Design review of the part built by this model. Coordinates are the model's own, in mm. A direction names the side the tool comes from. Round coordinates to 2 decimals unless told otherwise and drop trailing zeros. Write each loop counter-clockwise with the first axis right and the second up, starting at its lowest first coordinate (ties: lowest second). Pieces come first, ordered by that corner, then holes. Notation, with made-up numbers: (18.25, 45.5) -> (53.25, 45.5) arc R21 ccw to (53.25, 66.5) -> close; hole circle Ø9 at (45.5, 72). An arc over 180 degrees is marked (long way). Write item = value, one per line. Start each with the question number.
Item 1: To check wall thickness, follow L1, parallel to X at y = 1, z = -2.5; L2, parallel to X at y = 1.2, z = 18.5; L3, parallel to X at y = 12.5, z = 10.75. State the ranges of each line that lie inside material, in increasing order.
Item 2: Add section D-D, the plane z = 19. State the section outline as (x, y) points.
Item 3: Add section B-B, the plane x = 45.5. State the section outline as (y, z) points, then the cut area to 3 significant figures.
Item 4: For pin 1 Ø2.5 at (x, y) = (29, 4.5) entering from -Z; pin 2 Ø8 at (x, y) = (7, 13) entering from +Z; pin 3 Ø4 at (x, y) = (18, 3) entering from +Z; pin 4 Ø2 at (x, y) = (53.5, 3.5) entering from +Z, all flat-tipped, find the tip position at first contact; note any pin that passes through.
Item 5: Mouldability with a two-part tool opening along X and no side actions: class faces 1 (the cylindrical face through (-0.507, 12.187, 4.774)), 2 (the cylindrical face through (44.036, 0.986, -2.175)), 3 (the flat face through (51, 5.88, 8.08)) as released by +X, released by -X, zero draft, split by the parting line, or undercut.
Item 6: Add section A-A, the plane z = -2.5. State the section outline as (x, y) points, then the cut area to 3 significant figures.
Item 7: Add section C-C, the plane x = 29. State the section outline as (y, z) points, then the cut area to 3 significant figures.
Item 8: Machinability: for faces 4 (the flat face through (0, 1.9, 11.3)), 5 (the flat face through (3, 2, 17)), 6 (the flat face through (42, 1, -3)), 7 (the flat face through (47, 2, -1)), 8 (the cylindrical face through (56.916, 8.056, 7.409)), which of the approach directions +Z, -Z, +X, -X, +Y, -Y give a long, thin tool a straight path to every point of the face, cutting with its end or side? Answer none if there is none.
from build123d import *

# Parameters (mm, degrees)
SKETCH_1_W           = 50
SKETCH_1_H           = 16
EXTRUDE_1_DEPTH      = 15
SKETCH_2_W           = 8
SKETCH_2_H           = 5.2
SKETCH_2_R           = 1.5
EXTRUDE_2_DEPTH      = 2
FILLET_1_R           = 7
EXTRUDE_3_DEPTH      = 1
EXTRUDE_3_DEPTH_BACK = 51
SKETCH_3_R           = 6
EXTRUDE_4_DEPTH      = 12
EXTRUDE_4_DEPTH_BACK = 63
SKETCH_4_R           = 1.1


with BuildPart() as part:
    # Эскиз1 → Бобышка-Вытянуть1 (new body)
    with BuildSketch(Plane(origin=(0, 0, 0), x_dir=(1, 0, 0), z_dir=(0, 1, 0))):
        with Locations((25, -8)):
            Rectangle(SKETCH_1_W, SKETCH_1_H)
    extrude(amount=EXTRUDE_1_DEPTH)

    # Эскиз2 → Бобышка-Вытянуть2 (add)
    # profile 1 of 2: a face of its own
    with BuildSketch(Plane.XZ):
        with Locations((4, 18.6)):
            Rectangle(SKETCH_2_W, SKETCH_2_H)
        with Locations(Location((4.5, 18.5, 0), (0, 0, 270))):
            Circle(SKETCH_2_R, mode=Mode.SUBTRACT)
    # profile 2 of 2: a face of its own
    with BuildSketch(Plane.XZ):
        with Locations((46, -2.6)):
            Rectangle(SKETCH_2_W, SKETCH_2_H)
        with Locations(Location((45.5, -2.5, 0), (0, 0, 270))):
            Circle(SKETCH_2_R, mode=Mode.SUBTRACT)
    extrude(amount=-EXTRUDE_2_DEPTH)

    # Скругление1
    fillet_1_edges = [part.edges().sort_by_distance(p)[0] for p in [
        (25, 15, 0),
        (25, 15, 16),
    ]]
    fillet(fillet_1_edges, radius=FILLET_1_R)

    # Эскиз3 → Бобышка-Вытянуть3 (add, two sides: drawn at the far end of the back side and taken through both)
    with BuildSketch(Plane(origin=(50, 0, 0), x_dir=(0, 0, -1), z_dir=(1, 0, 0)).offset(-EXTRUDE_3_DEPTH_BACK)):
        with Locations((-8, 7.128166943)):
            Circle(SKETCH_3_R)
    extrude(amount=EXTRUDE_3_DEPTH + EXTRUDE_3_DEPTH_BACK)

    # Эскиз4 → Бобышка-Вытянуть4 (add, two sides: drawn at the far end of the back side and taken through both)
    with BuildSketch(Plane(origin=(51, 0, 0), x_dir=(0, 0, -1), z_dir=(1, 0, 0)).offset(-EXTRUDE_4_DEPTH_BACK)):
        with Locations((-8, 7.128166943)):
            Circle(SKETCH_4_R)
    extrude(amount=EXTRUDE_4_DEPTH + EXTRUDE_4_DEPTH_BACK)


solid = part.part
Result set:
q1.L1 = 42 to 44, 47 to 50
q1.L2 = 0 to 3, 6 to 8
q1.L3 = 0 to 50
q2.outline = (0, 0) -> (3.09, 0) -> (3.09, 2) -> (0, 2) -> close; (5.91, 0) -> (8, 0) -> (8, 2) -> (5.91, 2) -> close
q3.outline = (0, -5.2) -> (2, -5.2) -> (2, -4) -> (0, -4) -> close; (0, -1) -> (2, -1) -> (2, 0) -> (8, 0) arc R7 ccw to (15, 7) -> (15, 9) arc R7 ccw to (8, 16) -> (0, 16) -> close
q3.area = 223 mm²
q4.pin_1 = 0
q4.pin_2 = 15.93
q4.pin_3 = 16
q4.pin_4 = through
q5.face_1 = zero draft
q5.face_2 = undercut
q5.face_3 = released by +X
q6.outline = (42, 0) -> (44, 0) -> (44, 2) -> (42, 2) -> close; (47, 0) -> (50, 0) -> (50, 2) -> (47, 2) -> close
q6.area = 10.0 mm²
q7.outline = (0, 0) -> (8, 0) arc R7 ccw to (15, 7) -> (15, 9) arc R7 ccw to (8, 16) -> (0, 16) -> close
q7.area = 219 mm²
q8.face_4 = -X
q8.face_5 = +Z, +X, -X, +Y
q8.face_6 = -Z, -X, +Y, -Y
q8.face_7 = -Z, +X, -X, +Y
q8.face_8 = +X
